Part model, mm, in its own coordinate system. Face numbers are marked on the shaded views. Give positions to 0.01 mm unless a question says otherwise; leave off trailing zeros. Write each loop counter-clockwise with the first axis right and the second up, starting at its lowest first coordinate (ties: lowest second). Pieces come first, ordered by that corner, then holes. Notation, with made-up numbers: M -24.75,88.5 L 26.25,88.5 A21 ccw 26.25,117.5 Z; hole C -1.75,-16 d9. An arc over 180 degrees is marked long. Use a Markdown table: item, result.
```python
from build123d import *

# Parameters (mm, degrees)
F0_R     = 4.191
F1_DEPTH = 2.54


with BuildPart() as f1:
    # F0 (on Front) → F1 (new body)
    with BuildSketch(Plane.XZ):
        Polygon((-11.664975, 17.213106), (-11.664975, 11.244106), (-11.664975, 5.275106), (-5.969, 0), (0, 0), (5.969, 0), (11.424948, 5.0987), (11.424948, 11.0677), (11.424948, 17.0367), (5.969, 22.170171), (0, 22.170171), (-5.969, 22.170171), align=None)
        with Locations((0, 10.826342)):
            Circle(F0_R, mode=Mode.SUBTRACT)
    extrude(amount=F1_DEPTH)


solid = f1.part
```
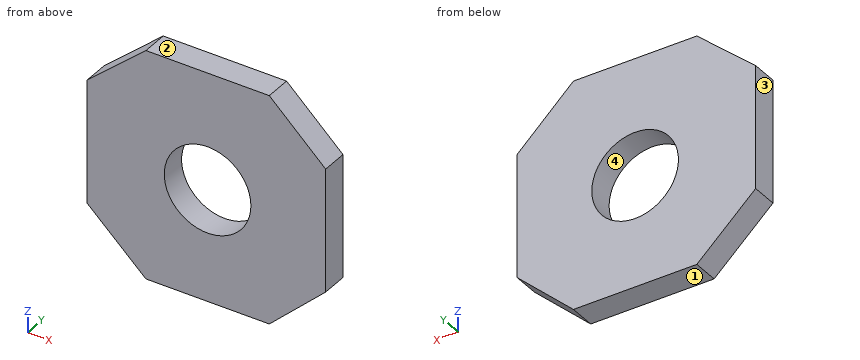
1. Cut at B-B, the plane z = 12.5. Give the cut face in (x, y), then the cut area to 3 significant figures.
Findings below:
| item | result |
|---|---|
| outline | M -11.66,-2.54 L -3.84,-2.54 L -3.84,0 L -11.66,0 Z; M 3.84,-2.54 L 11.42,-2.54 L 11.42,0 L 3.84,0 Z |
| area | 39.1 mm2 |
2. Cut at A-A, the plane x = 0. Give the cut face in (y, z).
Findings below:
| item | result |
|---|---|
| outline | M -2.54,0 L 0,0 L 0,6.64 L -2.54,6.64 Z; M -2.54,15.02 L 0,15.02 L 0,22.17 L -2.54,22.17 Z |
3. Two-plate mould, pull along Z, no slides. Class the marked faces 1, 2, 3 and 4: released by +Z, released by -Z, zero draft, split by the parting line, or undercut.
Findings below:
| item | result |
|---|---|
| face 1 | released by -Z |
| face 2 | released by +Z |
| face 3 | zero draft |
| face 4 | undercut |
4. Drill centre lines: L1, parallel to Z at x = 0, y = -1.7; L2, parallel to Z at x = -3.25, y = -0.15; L3, parallel to X at y = -0.4, z = 12.25. Where is each one in solid material? Low to high.
Findings below:
| item | result |
|---|---|
| L1 | 0 to 6.64, 15.02 to 22.17 |
| L2 | 0 to 8.18, 13.47 to 22.17 |
| L3 | -11.66 to -3.94, 3.94 to 11.42 |
5. Cut at C-C, the plane y = -1.3. Give the cut face in (x, z).
Findings below:
| item | result |
|---|---|
| outline | M -11.66,5.28 L -5.97,0 L 5.97,0 L 11.42,5.1 L 11.42,17.04 L 5.97,22.17 L -5.97,22.17 L -11.66,17.21 Z; hole C 0,10.83 d8.38 |
6. Drop flat-ended pins along their axis: P1, Ø1.5, axis at x = 9, y = -1, coming from the +Z side; P2, Ø5, axis at x = 0, z = 10.83, coming from the +Y side. Give the stop position or say it passes through.
Findings below:
| item | result |
|---|---|
| P1 | z = 20.02 |
| P2 | through |
7. Cut at D-D, the plane z = 18.5. Give the cut face in (x, y).
Findings below:
| item | result |
|---|---|
| outline | M -10.19,-2.54 L 9.87,-2.54 L 9.87,0 L -10.19,0 Z |
